Could you check a few things on this model? Use its own coordinates, in mm. Give positions to 0.01 mm unless a question says otherwise; leave off trailing zeros. Order: outer loops, then holes, each group sorted by start corner. A loop starts at its lowest first (then second) coordinate and runs counter-clockwise, first axis right, second up. Notation, with made-up numbers: (35, 83.25) - (69, 83.25) arc R25 ccw to (69, 116.25) - close; hole circle Ø2 at (-12.75, 82). An arc over 180 degrees is marked (long way). Put each result on its own line as item: value.
from build123d import *

# Parameters (mm, degrees)
SKETCH_R     = 2.5
SKETCH_R_2   = 1.5
PAD_DEPTH    = 3
SKETCH001_R  = 1.5
POCKET_DEPTH = 3.001


with BuildPart() as part:
    # Sketch → Pad (new body)
    with BuildSketch(Plane.XY):
        Polygon((0, 50), (0, 2), (-89, 2), (-91, 0), (-136, 0), (-139, 6), (-139, 36), (-137.020835, 38), (-100, 38), (-93, 50), align=None)
        with Locations((-133.6, 33.1)):
            Circle(SKETCH_R, mode=Mode.SUBTRACT)
        with Locations((-110.4, 33.1)):
            Circle(SKETCH_R, mode=Mode.SUBTRACT)
        with Locations((-110.4, 9.9)):
            Circle(SKETCH_R, mode=Mode.SUBTRACT)
        with Locations((-133.6, 9.9)):
            Circle(SKETCH_R, mode=Mode.SUBTRACT)
        with Locations((-90.5, 40)):
            Circle(SKETCH_R_2, mode=Mode.SUBTRACT)
        with Locations((-79.5, 40)):
            Circle(SKETCH_R_2, mode=Mode.SUBTRACT)
    pad = extrude(amount=PAD_DEPTH)

    # Mirrored: Pad across Sketch V_Axis
    add(pad.mirror(Plane(origin=(0, 0, 0), x_dir=(0, 0, 1), z_dir=(1, 0, 0))))

    # Sketch001 → Pocket (cut, through all)
    with BuildSketch(Plane.XY.offset(3)):
        with Locations((0, 32)):
            Circle(SKETCH001_R)
        with Locations((0, 10)):
            Circle(SKETCH001_R)
    extrude(amount=-POCKET_DEPTH, mode=Mode.SUBTRACT)


solid = part.part
1) We'd pull the mould along X, two halves only. Please class faces 1 (the flat face through (96.549, 43.916, 1.479)), 2 (the cylindrical face through (-136.1, 10, 1.5)), 3 (the flat face through (-2, 25, 0)): pulls with the +X half, pulls with the -X half, needs draft (parallel to the pull), parting line crosses it, or undercut.
Filled in:
face 1: pulls with the +X half
face 2: undercut
face 3: needs draft
2) Suppose I cut it at D-D, the plane y = 46.5. List the corners of the cut face in (x, z) for me, and give its area (3 significant figures).
Filled in:
outline: (-95.04, 0) - (95.04, 0) - (95.04, 3) - (-95.04, 3) - close
area: 570 mm^2
3) Suppose I cut it at A-A, the plane x = -110.4. List the corners of the cut face in (y, z) for me.
Filled in:
outline: (0, 0) - (7.4, 0) - (7.4, 3) - (0, 3) - close; (12.4, 0) - (30.6, 0) - (30.6, 3) - (12.4, 3) - close; (35.6, 0) - (38, 0) - (38, 3) - (35.6, 3) - close
4) Suppose I cut it at C-C, the plane x = -56. List the corners of the cut face in (y, z) for me, and give its area (3 significant figures).
Filled in:
outline: (2, 0) - (50, 0) - (50, 3) - (2, 3) - close
area: 144 mm^2
5) I'm going to push flat-ended pins straight in: pin 1 (6 mm diameter, centred on x = -133.6, y = 33.1, fed in from +Z); pin 2 (1.5 mm diameter, centred on x = 43.5, z = 1.5, fed in from -Y); pin 3 (0.9 mm diameter, centred on x = -121.5, z = 2, fed in from +Y). Where does each tip first touch, or does it pass through?
Filled in:
pin 1: stops at z = 3
pin 2: stops at y = 2
pin 3: stops at y = 38
6) If I drill on line 1 (Y direction, x = 0, z = 2.3); line 2 (Y direction, x = -110.4, z = 2.35); line 3 (X direction, y = 10.5, z = 2.05), over which ranges is the centre line in solid material (lowest first)? Write a range as [from, to].
Filled in:
line 1: y = [2, 8.5], [11.5, 30.5], [33.5, 50]
line 2: y = [0, 7.4], [12.4, 30.6], [35.6, 38]
line 3: x = [-139, -136.03], [-131.17, -112.83], [-107.97, -1.41], [1.41, 107.97], [112.83, 131.17], [136.03, 139]
7) Suppose I cut it at B-B, the plane z = 2.2. State how many separate pieces and enclosed holes the cut face has, and give its area (3 significant figures).
Filled in:
separate pieces: 1
enclosed holes: 14
area: 12,300 mm^2
